The listing builds one solid part. Answer for the finished solid, in the listing's coordinates (mm). Round coordinates to 2 decimals unless told otherwise and drop trailing zeros. Loops run counter-clockwise (first coordinate to the right, second up) from the corner with the lowest first, then second, coordinate; pieces in that order, holes last. Notation, with made-up numbers: (75, 27) -> (114, 27) arc R18 ccw to (114, 35) -> close; hole circle Ø1 at (-24, 85). An arc over 180 degrees is marked (long way). Use a Markdown table: item, result. Add a question column.
Q1. For a pull along X with two mould halves and no side action, classify faces 1 (the cylindrical face through (41.001, 167.86, 130.197)), 2 (the flat face through (2, 178, -2)), 3 (the cylindrical face through (23.73, 6.16, -75.35)) as released by +X, released by -X, zero draft, split by the parting line, or undercut.
Q2. Given pin 1 Ø2 at (x, z) = (65, 2) entering from -Y; pin 2 Ø8 at (y, z) = (149, -51.5) entering from -X; pin 3 Ø8 at (x, y) = (64.5, 92.5) entering from +Z, each flat-ended and moving along its own axis, determine where each tip first touches the part or whether it passes through.
Q3. Section C-C on y = 44.5 is taken. Give the vertices of the cut face in (x, z).
Q4. Section A-A on x = 0 is taken. Give the vertices of the cut face in (y, z).
Q5. Consider line 1 (Z direction, x = 0, y = 9.5); line 2 (Z direction, x = 0, y = 8.25); line 3 (X direction, y = 12, z = -39). Determine where each line is inside the solid, lowest interval first.
Q6. Section B-B on y = 66 is taken. Give the vertices of the cut face in (x, z).
from build123d import *

# Parameters (mm, degrees)
IZIM10_R                    = 136.5
IZIM9_R                     = 125
IZIM11_R                    = 136.5
Y_KSEKLIK_EKSTR_ZYON2_DEPTH = 20
IZIM12_R                    = 79
KES_EKSTR_ZYON3_DEPTH       = 12.5
KUBBE3_FACE_RADIUS          = 79
KUBBE3_HEIGHT               = 5


with BuildPart() as part:
    # Çizim10 → Loft2 section 0
    with BuildSketch(Plane(origin=(0, 158, 0), x_dir=(1, 0, 0), z_dir=(0, 1, 0))):
        Circle(IZIM10_R)
    # Çizim9 → Loft2 section 1
    with BuildSketch(Plane(origin=(0, 0, 0), x_dir=(1, 0, 0), z_dir=(0, 1, 0))):
        Circle(IZIM9_R)
    loft()

    # Çizim11 → Yükseklik-Ekstrüzyon2 (add)
    with BuildSketch(Plane(origin=(0, 158, 0), x_dir=(1, 0, 0), z_dir=(0, 1, 0))):
        with Locations(Location((0, 0, 0), (0, 0, 270))):
            Circle(IZIM11_R)
    extrude(amount=Y_KSEKLIK_EKSTR_ZYON2_DEPTH)

    # Çizim12 → Kes-Ekstrüzyon3 (cut)
    with BuildSketch(Plane.XZ):
        with Locations(Location((0, 0, 0), (0, 0, 270))):
            Circle(IZIM12_R)
    extrude(amount=-KES_EKSTR_ZYON3_DEPTH, mode=Mode.SUBTRACT)

    # Kubbe3: a dome of height H over a round flat face of radius A is a cap of a sphere of radius (A * A + H * H) / (2 * H)
    kubbe3_r = (KUBBE3_FACE_RADIUS * KUBBE3_FACE_RADIUS + KUBBE3_HEIGHT * KUBBE3_HEIGHT) / (2 * KUBBE3_HEIGHT)
    kubbe3_base = Plane((0, 12.5, 0), z_dir=(0, 1, 0))
    with Locations(kubbe3_base.offset(KUBBE3_HEIGHT - kubbe3_r)):
        kubbe3_ball = Sphere(kubbe3_r, mode=Mode.PRIVATE)
    add(split(kubbe3_ball, bisect_by=kubbe3_base, keep=Keep.TOP, mode=Mode.PRIVATE), mode=Mode.SUBTRACT)


solid = part.part
Checked values:
| question | item | result |
|---|---|---|
| 1 | face 1 | split by the parting line |
| 1 | face 2 | zero draft |
| 1 | face 3 | undercut |
| 2 | pin 1 | stops at y = 14.01 |
| 2 | pin 2 | stops at x = -127.3 |
| 2 | pin 3 | stops at z = 117.04 |
| 3 | outline | circle Ø256.48 at (0, 0) |
| 4 | outline | (0, -125) -> (158, -136.5) -> (178, -136.5) -> (178, 136.5) -> (158, 136.5) -> (0, 125) -> (0, 79) -> (12.5, 79) arc R626.6 cw to (12.5, -79) -> (0, -79) -> close |
| 5 | line 1 | z = -125.69 to -79, 79 to 125.69 |
| 5 | line 2 | z = -125.6 to -79, 79 to 125.6 |
| 5 | line 3 | x = -119.68 to -68.7, 68.7 to 119.68 |
| 6 | outline | circle Ø259.61 at (0, 0) |
